Input: part model. Units: mm. Frame: model coordinates. Face numbers are marked on the shaded views. A direction names the side the tool comes from. Coordinates: 2 decimals unless noted, no trailing zeros. Write each loop counter-clockwise with the first axis right and the second up, starting at its lowest first coordinate (ties: lowest second). Pieces come first, ordered by that corner, then holes. Notation, with made-up numbers: M -22.5,-7.75 L 2.5,-7.75 A22 cw 2.5,7.25 Z; hole C 14.5,-2.75 d9. An arc over 180 degrees is marked long. Answer as a JSON object with one key per item and string values. Group by question number.
from build123d import *

# Parameters (mm, degrees)
BOSS_EXTRUDE1_DEPTH = 5
BOSS_EXTRUDE2_DEPTH = 5
CUT_EXTRUDE3_START  = -5
CUT_EXTRUDE3_DEPTH  = 5
SKETCH4_W           = 3
SKETCH4_H           = 4
BOSS_EXTRUDE3_DEPTH = 5
SKETCH5_W           = 1
SKETCH5_H           = 3
CUT_EXTRUDE4_DEPTH  = 5


# Read off the part's stored shape, not the designer's step: Cut-Extrude3
with BuildPart() as part:
    # Sketch1 → Boss-Extrude1 (new body)
    with BuildSketch(Plane.XY):
        with BuildLine():
            add(Edge.make_bspline(
                [(-5, 0), (-1.114165851, -7.611100797), (-10, -11.5)],
                knots=[0, 0, 0, 1, 1, 1], degree=2))
            Line((-10, -11.5), (-13, -11.5))
            Line((-13, -11.5), (-13, -8.5))
            Line((-13, -8.5), (-16, -8.5))
            Line((-16, -8.5), (-16, -11.5))
            Line((-16, -11.5), (-19, -11.5))
            Line((-19, -11.5), (-19, -8.5))
            Line((-19, -8.5), (-22, -8.5))
            Line((-22, -8.5), (-22, -15.5))
            Line((-22, -15.5), (-17.468951593, -15.5))
            add(Edge.make_bspline(
                [(-17.468951593, -15.5), (-11.464221473, -17.002032437), (-4.91520191, -15.903447496), (0.325280881, -12.931109156)],
                knots=[0.25236579, 0.25236579, 0.25236579, 0.25236579, 1.015713885, 1.015713885, 1.015713885, 1.015713885], degree=3))
            ThreePointArc((0.325280881, -12.931109156), (2.765522994, -9.541735665), (1.782110459, -5.482729135))
            Line((1.782110459, -5.482729135), (-1.569443242, -1.2396967))
            ThreePointArc((-1.569443242, -1.2396967), (-1.2396967, 1.569443242), (1.569443242, 1.2396967))
            Line((1.569443242, 1.2396967), (3.215278379, -0.843913615))
            ThreePointArc((3.215278379, -0.843913615), (4.328084119, -1.168713777), (5, -0.224065265))
            Line((5, -0.224065265), (5, 0.290683459))
            ThreePointArc((5, 0.290683459), (3.541503697, 3.541503697), (0.290683459, 5))
            Line((0.290683459, 5), (0, 5))
            ThreePointArc((0, 5), (-3.535533906, 3.535533906), (-5, 0))
        make_face()
    extrude(amount=BOSS_EXTRUDE1_DEPTH)

    # Sketch2 → Boss-Extrude2 (add)
    with BuildSketch(Plane.XY.offset(5)):
        with BuildLine():
            Line((2.189291593, 0.454975079), (2.809139943, -0.329746542))
            ThreePointArc((2.809139943, -0.329746542), (2.106854957, -0.247309907), (2.189291593, 0.454975079))
        make_face()
        with BuildLine():
            Line((-0.329746542, -2.809139943), (-0.949594892, -2.024418322))
            ThreePointArc((-0.949594892, -2.024418322), (-0.247309907, -2.106854957), (-0.329746542, -2.809139943))
        make_face()
    extrude(amount=-BOSS_EXTRUDE2_DEPTH)

    # Cut-Extrude3 outline → Cut-Extrude3 (cut)
    with BuildSketch(Plane.XY.offset(5).offset(CUT_EXTRUDE3_START)):
        with BuildLine():
            add(Edge.make_bspline(
                [(-4.271989908, -1.710772943), (-2.750457375, -4.583809325), (2.811238363, -9.068198313), (-7.188128971, -13.02856833), (-10, -11.5)],
                knots=[0.076818774, 0.076818774, 0.076818774, 0.076818774, 0.487236237, 1, 1, 1, 1], degree=3))
            add(Edge.make_bspline(
                [(-4.271989908, -1.710772943), (-2.141880314, -8.060881638), (-10, -11.5)],
                knots=[0.115657624, 0.115657624, 0.115657624, 1, 1, 1], degree=2))
        make_face()
    extrude(amount=CUT_EXTRUDE3_DEPTH, mode=Mode.SUBTRACT)

    # Sketch4 → Boss-Extrude3 (add)
    with BuildSketch(Plane.XY.offset(5)):
        with Locations((-23.5, -13.5)):
            Rectangle(SKETCH4_W, SKETCH4_H)
        with BuildLine():
            Line((-22, -8.5), (-19, -8.5))
            ThreePointArc((-19, -8.5), (-18.75, -8.25), (-19, -8))
            Line((-19, -8), (-22, -8))
            ThreePointArc((-22, -8), (-22.25, -8.25), (-22, -8.5))
        make_face()
        with BuildLine():
            Line((-16, -8.5), (-13, -8.5))
            ThreePointArc((-13, -8.5), (-12.75, -8.25), (-13, -8))
            Line((-13, -8), (-16, -8))
            ThreePointArc((-16, -8), (-16.25, -8.25), (-16, -8.5))
        make_face()
    extrude(amount=-BOSS_EXTRUDE3_DEPTH)

    # Sketch5 → Cut-Extrude4 (cut)
    with BuildSketch(Plane.XY.offset(5)):
        with Locations((-20.5, -9.5)):
            Rectangle(SKETCH5_W, SKETCH5_H)
        with Locations((-14.5, -9.5)):
            Rectangle(SKETCH5_W, SKETCH5_H)
    extrude(amount=-CUT_EXTRUDE4_DEPTH, mode=Mode.SUBTRACT)


solid = part.part
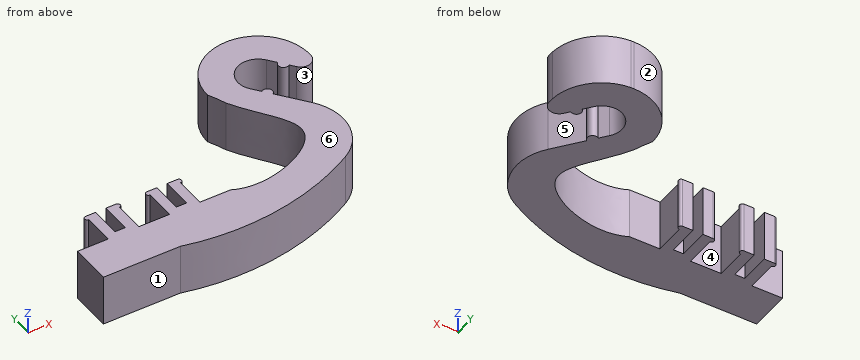
Q1. Section C-C, the plane y = 3.75. Return the cut outline in (x, z), and give its area (3 significant figures).
Q2. Section A-A, the plane x = 1. Return the cut outline in (y, z).
Q3. Draft query along X for the marked faces 1, 2 and 3. Return one class per face: released by +X, released by -X, zero draft, split by the parting line, or undercut.
Q4. Line query: line 1 (X direction, y = -10, z = 1.7); line 2 (Y direction, x = -18.5, z = 1.35); line 3 (Y direction, x = -11.5, z = 4.15). Output: solid intervals per line, ascending. Write a range as from..to.
Q5. Section B-B, the plane y = -10. State how many separate pieces and enclosed holes the cut face has, and give its area (3 significant figures).
Q6. Access query for the marked faces 4, 5 and 6. Directions: +Z, -Z, +X, -X, +Y, -Y. A direction counts if a zero-diameter tool reaches every point of the face in a straight line with its end or side. Return the directions, or none.
Q7. Pin query (flat end, axial travel): pin 1 Ø2 at (x, z) = (-15.5, 3.5) entering from +Y; pin 2 Ø1.5 at (y, z) = (-10, 3.5) entering from +X; pin 3 Ø0.9 at (x, z) = (-23, 2) entering from +Y. Return the tip coordinate at first contact, or that it passes through.
Filled in:
{
 "1": {"outline": "M -3.31,0 L 3.32,0 L 3.32,5 L -3.31,5 Z", "area": "33.1 mm^2"},
 "2": {"outline": "M -12.47,0 L -4.49,0 L -4.49,5 L -12.47,5 Z; M 1.73,0 L 4.91,0 L 4.91,5 L 1.73,5 Z"},
 "3": {"face 1": "zero draft", "face 2": "released by -X", "face 3": "undercut"},
 "4": {"line 1": "-22..-21, -20..-19, -16..-15, -14..-13, -2.04..2.65", "line 2": "-15.5..-11.5", "line 3": "-16.17..-11.5"},
 "5": {"separate pieces": "5", "enclosed holes": "0", "area": "43.5 mm^2"},
 "6": {"face 4": "+Z, -Z", "face 5": "+Z, -Z, +X", "face 6": "+Z, +X, -X, +Y, -Y"},
 "7": {"pin 1": "y = -8", "pin 2": "x = 2.81", "pin 3": "y = -11.5"}
}
